Input: part model. Units: mm. Frame: model coordinates. A direction names the side the tool comes from. Give positions to 0.01 mm unless a question says otherwise; leave off trailing zeros. Loops run counter-clockwise (first coordinate to the right, second up) from the corner with the lowest first, then second, coordinate; pieces in that order, holes last. Notation, with made-up numbers: M -19,24 L 18,24 A22 cw 18,55 Z; hole C -13,84.5 d9. An arc over 180 degrees is marked long. Answer as a JSON object with one key per item and string values. Group by question number.
```python
from build123d import *

# Parameters (mm, degrees)
BOSS_EXTRUDE1_DEPTH = 75
CUT_EXTRUDE1_DEPTH  = 72.5
SKETCH6_W           = 30
SKETCH6_H           = 2.5
SKETCH6_W_2         = 2.5
SKETCH6_H_2         = 30
CUT_EXTRUDE4_DEPTH  = 2.5
SKETCH8_R           = 5
CUT_EXTRUDE5_DEPTH  = 5


with BuildPart() as part:
    # Sketch1 → Boss-Extrude1 (new body)
    with BuildSketch(Plane.XY):
        Polygon((0, 0), (170, 0), (170, 135), (145.104076401, 195.104076401), (85, 220), (24.895923599, 195.104076401), (0, 135), align=None)
    extrude(amount=BOSS_EXTRUDE1_DEPTH)

    # Sketch2 → Cut-Extrude1 (cut)
    with BuildSketch(Plane.XY.offset(75)):
        Polygon((167.5, 134.502719082), (143.190659239, 193.190659239), (85, 217.294019499), (26.809340761, 193.190659239), (2.5, 134.502719082), (2.5, 2.5), (167.5, 2.5), align=None)
    extrude(amount=-CUT_EXTRUDE1_DEPTH, mode=Mode.SUBTRACT)

    # Sketch6 → Cut-Extrude4 (cut)
    with BuildSketch(Plane.XY.offset(75)):
        with Locations((135, 1.25)):
            Rectangle(SKETCH6_W, SKETCH6_H)
        with Locations((168.75, 35)):
            Rectangle(SKETCH6_W_2, SKETCH6_H_2)
        Polygon((101.616080276, 210.411413695), (129.332466251, 198.930910725), (130.289174832, 201.240609556), (102.572788857, 212.721112527), align=None)
        with Locations((168.75, 95)):
            Rectangle(SKETCH6_W_2, SKETCH6_H_2)
        Polygon((67.427211143, 212.721112527), (68.383919724, 210.411413695), (40.667533749, 198.930910725), (39.710825168, 201.240609556), align=None)
        with Locations((1.25, 95)):
            Rectangle(SKETCH6_W_2, SKETCH6_H_2)
        with Locations((1.25, 35)):
            Rectangle(SKETCH6_W_2, SKETCH6_H_2)
        with Locations((35, 1.25)):
            Rectangle(SKETCH6_W, SKETCH6_H)
    extrude(amount=-CUT_EXTRUDE4_DEPTH, mode=Mode.SUBTRACT)

    # Sketch8 → Cut-Extrude5 (cut)
    with BuildSketch(Plane(origin=(0, 2.5, 0), x_dir=(1, 0, 0), z_dir=(0, 1, 0))):
        with Locations((150, -40)):
            Circle(SKETCH8_R)
    extrude(amount=-CUT_EXTRUDE5_DEPTH, mode=Mode.SUBTRACT)


solid = part.part
```
1. Section A-A (z = 60). Output: boundary loops of the cut face in (x, y).
2. Mould query, pull axis Z, two halves, no side actions, for faces 1 (the flat face through (116, 206, 72.5)), 2 (the flat face through (84, 112, 0)), 3 (the flat face through (2.5, 69, 39)), 4 (the cylindrical face through (145, 1, 40)). Classes: pulls with the +Z half, pulls with the -Z half, needs draft (parallel to the pull), parting line crosses it, or undercut.
3. Section C-C (z = 40). Output: boundary loops of the cut face in (x, y).
4. Section D-D (x = 115.5). Output: boundary loops of the cut face in (y, z), then the cut area to 3 significant figures.
5. First-contact query: P1, Ø0.8, axis at y = 2, z = 73.5, coming from the -X side; P2, Ø3, axis at x = 139, y = 0.5, coming from the +Z side; P3, Ø10, axis at x = 36, y = 78, coming from the +Z side; P4, Ø2, axis at x = 1, z = 74, coming from the +Y side. Flat tips, straight axial feed; report the tip coordinate or a pass-through.
6. Reachability of faces 5 (the flat face through (84, 111, 2.5)), 6 (the flat face through (12.62, 165.47, 36.98)) from +Z, -Z, +X, -X, +Y, -Y: full face, straight path, thin tool, end or side. Return the list, or none.
7. Material intervals for L1, parallel to X at y = 1.8, z = 40; L2, parallel to X at y = 111.5, z = 21; L3, parallel to Z at x = 102.5, y = 199, sorted ascending.
8. Section B-B (x = 61). Output: boundary loops of the cut face in (y, z), then the cut area to 3 significant figures.
Geometry results:
{
 "1": {"outline": "M 0,0 L 170,0 L 170,135 L 145.1,195.1 L 85,220 L 24.9,195.1 L 0,135 Z; hole M 2.5,2.5 L 167.5,2.5 L 167.5,134.5 L 143.19,193.19 L 85,217.29 L 26.81,193.19 L 2.5,134.5 Z"},
 "2": {"face 1": "pulls with the +Z half", "face 2": "pulls with the -Z half", "face 3": "needs draft", "face 4": "undercut"},
 "3": {"outline": "M 0,0 L 145,0 L 145,2.5 L 2.5,2.5 L 2.5,134.5 L 26.81,193.19 L 85,217.29 L 143.19,193.19 L 167.5,134.5 L 167.5,2.5 L 155,2.5 L 155,0 L 170,0 L 170,135 L 145.1,195.1 L 85,220 L 24.9,195.1 L 0,135 Z"},
 "4": {"outline": "M 0,0 L 207.37,0 L 207.37,72.5 L 204.66,72.5 L 204.66,2.5 L 2.5,2.5 L 2.5,75 L 0,75 Z", "area": "889 mm2"},
 "5": {"P1": "x = 0", "P2": "z = 72.5", "P3": "z = 2.5", "P4": "y = 139.83"},
 "6": {"face 5": "+Z", "face 6": "+Z, -Z, -X, +Y"},
 "7": {"L1": "0 to 145, 155 to 170", "L2": "0 to 2.5, 167.5 to 170", "L3": "0 to 2.5"},
 "8": {"outline": "M 0,0 L 210.06,0 L 210.06,72.5 L 207.35,72.5 L 207.35,2.5 L 2.5,2.5 L 2.5,75 L 0,75 Z", "area": "896 mm2"}
}
